from build123d import *

# Parameters (mm, degrees)
BOSS_EXTRUDE1_DEPTH                               = 6.35
BOSS_EXTRUDE2_DEPTH                               = 6.35
CSK_FOR_8_FLAT_HEAD_MACHINE_SCREW_100_D           = 4.9149
CSK_FOR_8_FLAT_HEAD_MACHINE_SCREW_100_DEPTH       = 6.35
CSK_FOR_8_FLAT_HEAD_MACHINE_SCREW_100_CSINK_D     = 8.4328
CSK_FOR_8_FLAT_HEAD_MACHINE_SCREW_100_CSINK_ANGLE = 100


with BuildPart() as part:
    # Sketch1 → Boss-Extrude1 (new body)
    with BuildSketch(Plane.XY):
        Polygon((2683.510000011, 6621.1958), (2683.510000013, 5955.03), (2911.730002065, 5955.03), (2911.730002065, 5935.980000183), (2962.998658572, 5935.980000183), (3014.728804207, 5957.938144244), (2987.930002065, 6744.189464503), align=None)
    extrude(amount=BOSS_EXTRUDE1_DEPTH)

    # Sketch2 → Boss-Extrude2 (add)
    with BuildSketch(Plane.XY.offset(6.35)):
        Polygon((2933.697739453, 6621.1958), (2683.510000011, 6621.1958), (2683.510000386, 6602.1458), (2933.697739453, 6602.1458), align=None)
    extrude(amount=-BOSS_EXTRUDE2_DEPTH)

    # CSK for #8 Flat Head Machine Screw (100)2
    with Locations(Plane.XY.offset(6.35)):
        with Locations((2871.150804655, 6611.6708), (2746.056935059, 6611.6708), (2746.056934863, 6440.805), (2871.15080459, 6440.805), (2746.0569351, 6275.705000214), (2871.150804763, 6275.705000214), (2944.446214291, 5945.505000556), (2996.439588076, 6026.795207351), (2985.802221481, 6331.409531427), (2983.142879832, 6407.563112446), (2980.483538184, 6483.716693465), (2977.824196535, 6559.870274483), (2975.164854886, 6636.023855502), (2972.505513237, 6712.177436521)):
            CounterSinkHole(CSK_FOR_8_FLAT_HEAD_MACHINE_SCREW_100_D / 2, CSK_FOR_8_FLAT_HEAD_MACHINE_SCREW_100_CSINK_D / 2, depth=CSK_FOR_8_FLAT_HEAD_MACHINE_SCREW_100_DEPTH, counter_sink_angle=CSK_FOR_8_FLAT_HEAD_MACHINE_SCREW_100_CSINK_ANGLE)


solid = part.part
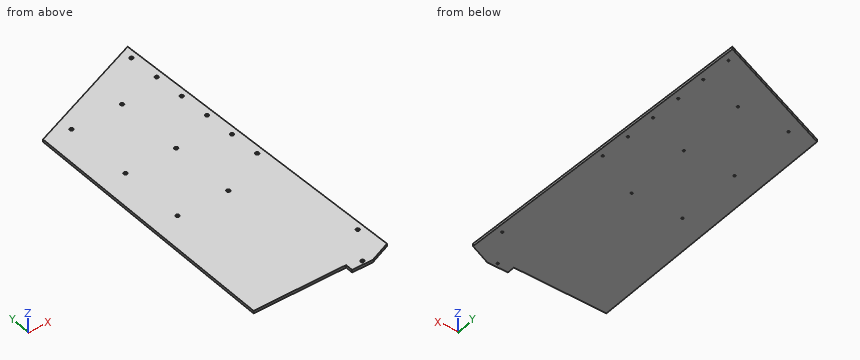
Could you check a few things on this model? Use its own coordinates, in mm. Give positions to 0.01 mm unless a question says otherwise; leave off trailing zeros. Order: outer loops, then holes, each group sorted by start corner. A loop starts at its lowest first (then second) coordinate and runs counter-clockwise, first axis right, second up.
Item 1: If we section it at C-C, the plane x = 2823: Write out the boundary of the cut face in (y, z), plus the area to 3 significant figures.
Item 2: I need wall thicknesses on line 1 (X direction, y = 6366, z = 0.5); line 2 (X direction, y = 6214.5, z = 6.25); line 3 (Y direction, x = 2734.5, z = 4.5). Which ranges of each line are inside material? Lowest first, please.
Item 3: If we section it at A-A, the plane z = 1: Count the separate pieces of the cut face and the enclosed holes in it, plus the area to 3 significant figures.
Item 4: If we section it at B-B, the plane y = 6312.5: Write out the boundary of the cut face in (x, z), plus the area to 3 significant figures.
Item 5: I'm going to push flat-ended pins straight in: pin 1 (3 mm diameter, centred on x = 2985.8, y = 6331.41, fed in from -Z); pin 2 (6.5 mm diameter, centred on x = 2746.06, y = 6611.67, fed in from +Z); pin 3 (8 mm diameter, centred on x = 2972.51, y = 6712.18, fed in from +Z); pin 4 (1.9 mm diameter, centred on x = 2755, z = 3, fed in from -Y). Where does each tip first touch, or does it pass through?
Values:
1. outline: (5955.03, 0) - (6677.55, 0) - (6677.55, 6.35) - (5955.03, 6.35) - close
1. area: 4,590 mm2
2. line 1: x = 2683.51 to 3000.82
2. line 2: x = 2683.51 to 3005.98
2. line 3: y = 5955.03 to 6641.8
3. separate pieces: 1
3. enclosed holes: 14
3. area: 233,000 mm2
4. outline: (2683.51, 0) - (3002.64, 0) - (3002.64, 6.35) - (2683.51, 6.35) - close
4. area: 2,030 mm2
5. pin 1: passes through
5. pin 2: stops at z = 5.54
5. pin 3: stops at z = 6.17
5. pin 4: stops at y = 5955.03
